Verification items for the finished model (mm, model axes). A direction names the side the tool comes from. Coordinates: 2 decimals unless noted, no trailing zeros. Write each loop counter-clockwise with the first axis right and the second up, starting at its lowest first coordinate (ties: lowest second). Pieces come first, ordered by that corner, then holes. Notation, with made-up numbers: (88, 81.5) -> (108, 81.5) arc R14 cw to (108, 87.5) -> close; hole circle Ø1 at (85.25, -9). An arc over 180 degrees is marked (long way). Write item = value, one per line. Start each with the question number.
(1) Section check C-C (x = 55). Record the cut outline in (y, z), plus the area to 3 significant figures.
(2) Mould release check, pull along X, two halves, no side actions. Record for faces 5 (the face through (21, 0, 42)), 6 (the face through (30, 20, 15)), 7 (the face through (46, 38, 62)), 8 (the face through (20, 40, 15)): released by +X, released by -X, zero draft, split by the parting line, or undercut.
(3) Material ranges on probe 1 along Z at (x, y) = (60.5, 37); probe 2 along Z at (x, y) = (-10, 5); probe 3 along X at (y, z) = (15.5, 14), recorded low to high. Write a range as [from, to].
(4) Section check B-B (y = 91). Record the cut outline in (x, z), plus the area to 3 significant figures.
(5) Section check D-D (z = 40.5). Record the cut outline in (x, y), plus the area to 3 significant figures.
(6) Section check A-A (z = 18.5). Record the cut outline in (x, y), plus the area to 3 significant figures.
(7) Gauge pin test, flat ends, axial feed: pin 1 Ø5 at (x, z) = (70, 6) entering from -Y; pin 2 Ø11 at (y, z) = (33.5, 2.5) entering from -X; pin 3 Ø22 at (y, z) = (71, 72.5) entering from +X. Record the tip position at first contact, or that the pin passes through.
(8) Set-up check for faces 1 (the face through (5, 49, 85)), 2 (the face through (65, 25, 5)), 3 (the face through (50, 89, 71)), 4 (the face through (20, 20, 30)): record each of +Z, -Z, +X, -X, +Y, -Y from which the full face is reachable in a straight line by a thin tool's end or side.
```python
from build123d import *

# Parameters (mm, degrees)
F0_W          = 100
F0_H          = 85
F1_DEPTH      = 75
F1_DEPTH_BACK = 25
F3_DEPTH      = 100
F4_W          = 20
F4_H          = 30
F5_DEPTH      = 40
F7_DEPTH      = 100
F8_W          = 10
F8_H          = 50
F9_DEPTH      = 25
F16_DEPTH     = 25


with BuildPart() as f1:
    # F0 (on Right) → F1 (new body, two sides)
    with BuildSketch(Plane.YZ) as f1_sk:
        with Locations((50, 42.5)):
            Rectangle(F0_W, F0_H)
    extrude(amount=F1_DEPTH)
    extrude(f1_sk.sketch, amount=-F1_DEPTH_BACK)

    # F2 (on Front) → F3 (cut, through all)
    with BuildSketch(Plane.XZ):
        Polygon((0, 10), (-25, 60), (-25, 0), (0, 0), align=None)
    extrude(amount=-F3_DEPTH, mode=Mode.SUBTRACT)

    # F4 (on Front) → F5 (cut)
    with BuildSketch(Plane.XZ):
        with Locations((20, 15)):
            Rectangle(F4_W, F4_H)
    extrude(amount=-F5_DEPTH, mode=Mode.SUBTRACT)

    # F6 (on Front) → F7 (cut, through all)
    with BuildSketch(Plane.XZ):
        Polygon((60, 65), (60, 10), (75, 10), (75, 85), (50, 85), (50, 65), align=None)
    extrude(amount=-F7_DEPTH, mode=Mode.SUBTRACT)

    # F8 (on Top) → F9 (cut)
    with BuildSketch(Plane.XY):
        with Locations((70, 25)):
            Rectangle(F8_W, F8_H)
    extrude(amount=F9_DEPTH, mode=Mode.SUBTRACT)

    # F15 (on 3pt) → F16 (cut)
    with BuildSketch(Plane(origin=(51.4285714286, -12.8571428571, 25.7142857143), x_dir=(0.1951800146, 0.9759000729, 0.0975900073), z_dir=(0.8728715609, -0.2182178902, 0.4364357805))):
        Polygon((95.1502571125, 55.9016994375), (84.9033063465, 57.0197334262), (35.3343970406, 62.4281448313), (13.1746509848, 64.8459713475), (13.1746509848, -13.416407865), (115.6441586444, 31.304951685), (74.6563555806, 35.77708764), (115.6441586444, 53.66563146), align=None)
    extrude(amount=F16_DEPTH, mode=Mode.SUBTRACT)


solid = f1.part
```
Response:
q1.outline = (0, 0) -> (100, 0) -> (100, 65) -> (80, 65) -> (0, 25) -> close
q1.area = 4,900 mm2
q2.face_5 = zero draft
q2.face_6 = undercut
q2.face_7 = released by +X
q2.face_8 = undercut
q3.probe_1 = [0, 10]
q3.probe_2 = [30, 85]
q3.probe_3 = [-2, 10], [30, 60]
q4.outline = (-25, 60) -> (0, 10) -> (0, 0) -> (75, 0) -> (75, 10) -> (60, 10) -> (60, 60.5) -> (57.75, 65) -> (50, 65) -> (50, 80.5) -> (47.75, 85) -> (-25, 85) -> close
q4.area = 6,290 mm2
q5.outline = (-15.25, 0) -> (47.25, 0) -> (60, 51) -> (60, 100) -> (-15.25, 100) -> close
q5.area = 7,200 mm2
q6.outline = (-4.25, 0) -> (10, 0) -> (10, 40) -> (30, 40) -> (30, 0) -> (58.25, 0) -> (60, 7) -> (60, 100) -> (-4.25, 100) -> close
q6.area = 5,620 mm2
q7.pin_1 = 50
q7.pin_2 = 0
q7.pin_3 = 55.15
q8.face_1 = +Z, +X, -X, +Y, -Y
q8.face_2 = +Z, -Z, +X, -Y
q8.face_3 = +Z, +X, +Y, -Y
q8.face_4 = -Z, -Y
